Model file for the job. Use its own axes, mm. Face numbers are marked on the shaded views. A direction names the side the tool comes from. Coordinates: 2 decimals unless noted, no trailing zeros. Write each loop counter-clockwise with the first axis right and the second up, starting at its lowest first coordinate (ties: lowest second). Pieces come first, ordered by that corner, then holes. Notation, with made-up numbers: (70, 48.25) - (109, 48.25) arc R21 ccw to (109, 60.25) - close; hole circle Ø6 at (43.5, 37). An arc over 180 degrees is marked (long way). Put each result on its own line as item: value. Start each with the question number.
1. Which spindle directions (+Z, -Z, +X, -X, +Y, -Y) get a long thin tool onto all of the face, cutting with end or side? Do the marked faces 4 and 5. Say none if no direction does.
2. Pull direction X, two halves, no side cores. Call the marked faces 1, 2 and 3: released by +X, released by -X, zero draft, split by the parting line, or undercut.
3. Drill centre lines: L1, parallel to Y at x = 0, z = -57.75; L2, parallel to Y at x = 0, z = 4.75; L3, parallel to Z at x = 0, y = -20 (3 decimals). Where is each one in solid material? Low to high. Write a range as from..to.
4. Saw through at D-D, the plane y = -6.5. Write the cut outline in (x, z).
5. Saw through at C-C, the plane z = -5.5. Write the cut outline in (x, y), plus the area to 3 significant figures.
6. Drop flat-ended pins along their axis: P1, Ø6, axis at y = -9.5, z = -4, coming from the +X side; P2, Ø12, axis at x = -7.5, z = -34.5, coming from the -Y side; P3, Ø4, axis at x = 8, y = -1, coming from the +Z side. Give the stop position or say it passes through.
7. Saw through at A-A, the plane y = 0. Write the cut outline in (x, z).
8. Saw through at B-B, the plane x = 5.5. Write the cut outline in (y, z), plus the area to 3 significant figures.
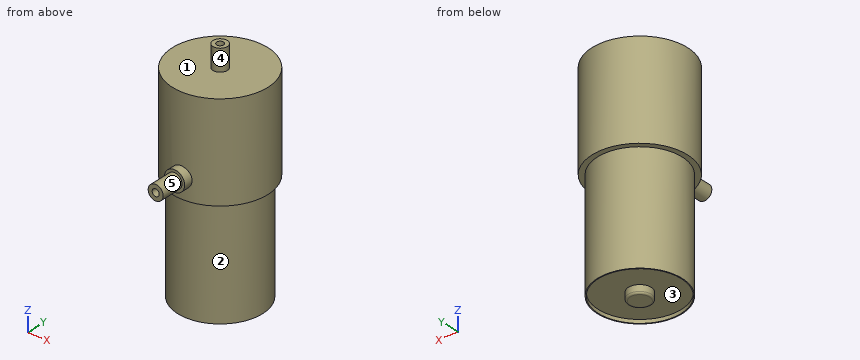
Autodesk Inventor part; units mm, degrees
ref_plane "Work Plane1" through (0, -13.5, 0) normal (0, 1, 0) x (-1, 0, 0)
ref_plane "YZ Plane" through (0, 0, 0) normal (1, 0, 0) x (0, 1, 0)
ref_plane "XY Plane" through (0, 0, 0) normal (0, 0, 1) x (1, 0, 0)
sketch "Sketch1" plane through (0, 0, 0) normal (0, 0, 1) x (1, 0, 0)
  circle A0 centre (0, 0) radius 13.5
  circle A1 centre (0, 0) radius 2.05
  circle A2 centre (0, 0) radius 12
  circle A3 centre (0, 0) radius 1
  dimension "d0" = 27
  dimension "d3" = 4.1
  dimension "d6" = 24
  dimension "d20" = 2
extrude "Extrusion1" add sketch "Sketch1" against normal blind 27.3 contours A0 | A1 | A2 | A3
extrude "Extrusion2" add sketch "Sketch1" along normal blind 6.1 contours A1 | A3
extrude "Extrusion3" add sketch "Sketch1" against normal blind 58.2 contours A1 | A2 | A3
ref_plane "Work Plane1" through (0, -13.5, 0) normal (0, 1, 0) x (-1, 0, 0)
sketch "Sketch2" plane through (0, -13.5, 0) normal (0, 1, 0) x (-1, 0, 0)
  circle A0 centre (0, -21.675) radius 2.875
  circle A1 centre (0, -21.675) radius 2.125
  line L0 (13.5, 0) -> (-13.5, 0)
  circle A2 centre (0, -21.675) radius 1
  point P0 (0, 0)
  dimension "d10" = 5.75
  dimension "d11" = 21.675
  dimension "d12" = 4.25
  dimension "d17" = 2
extrude "Extrusion4" add sketch "Sketch2" along normal mid plane 4.5 contours A0 | A1 | A2
extrude "Extrusion5" add sketch "Sketch2" against normal blind 8.75 contours A1 | A2
extrude "Extrusion6" cut sketch "Sketch2" against normal through all contours A2
extrude "Extrusion7" cut sketch "Sketch1" along normal through all contours A3
sketch "Sketch3" plane through (0, 0, -58.2) normal (0, 0, -1) x (-1, 0, 0)
  circle A0 centre (0, 0) radius 3.25
  circle A1 centre (0, 0) radius 11.75
  dimension "d23" = 6.5
  dimension "d26" = 23.5
extrude "Extrusion9" cut sketch "Sketch3" against normal blind 1
extrude "Extrusion10" add sketch "Sketch3" along normal blind 1.25 contours A0
fillet "Fillet1" radius 0.5 1 edges at (3.25, 0, -59.45)
equation "\"d9\" = -0.5 * d0"
properties part number "Adafruit_1528_4699_ND"
Final values:
1. face 4: +Z
1. face 5: -Y
2. face 1: zero draft
2. face 2: split by the parting line
2. face 3: undercut
3. L1: y = -12..-11.75, -3.25..3.25, 11.75..12
3. L2: y = -2.05..-1, 1..2.05
3. L3: z = -23.8..-22.675, -20.675..-19.55
4. outline: (-11.83, -27.3) - (-10.09, -27.3) - (-10.09, -58.2) - (-9.79, -58.2) - (-9.79, -57.2) - (9.79, -57.2) - (9.79, -58.2) - (10.09, -58.2) - (10.09, -27.3) - (11.83, -27.3) - (11.83, 0) - (-11.83, 0) - close
5. outline: circle Ø27 at (0, 0)
5. area: 573 mm²
6. P1: stops at x = 11.83
6. P2: stops at y = -11.91
6. P3: stops at z = 0
7. outline: (-13.5, -27.3) - (-12, -27.3) - (-12, -58.2) - (-11.75, -58.2) - (-11.75, -57.2) - (-3.25, -57.2) - (-3.25, -58.95) arc R0.5 ccw to (-2.75, -59.45) - (2.75, -59.45) arc R0.5 ccw to (3.25, -58.95) - (3.25, -57.2) - (11.75, -57.2) - (11.75, -58.2) - (12, -58.2) - (12, -27.3) - (13.5, -27.3) - (13.5, 0) - (2.05, 0) - (2.05, 6.1) - (1, 6.1) - (1, 0) - (-1, 0) - (-1, 6.1) - (-2.05, 6.1) - (-2.05, 0) - (-13.5, 0) - close
8. outline: (-12.33, -27.3) - (-10.67, -27.3) - (-10.67, -58.2) - (-10.38, -58.2) - (-10.38, -57.2) - (10.38, -57.2) - (10.38, -58.2) - (10.67, -58.2) - (10.67, -27.3) - (12.33, -27.3) - (12.33, 0) - (-12.33, 0) - close
8. area: 1,310 mm²
